```python
from build123d import *

# Parameters (mm, degrees)
F0_R     = 15
F0_R_2   = 5
F0_R_3   = 25
F1_DEPTH = 25


with BuildPart() as f1:
    # F0 (on Top) → F1 (new body)
    with BuildSketch(Plane.XY):
        with BuildLine():
            Line((-70.938008, -68.265357), (-67.75825, -73.265357))
            Line((-67.75825, -73.265357), (45.419062, -73.265357))
            Line((45.419062, -73.265357), (49.061992, -68.265357))
            Line((49.061992, -68.265357), (49.061992, -53.265357))
            Line((49.061992, -53.265357), (89.061992, -53.265357))
            Line((89.061992, -53.265357), (89.061992, 21.734643))
            ThreePointArc((89.061992, 21.734643), (81.739661, 39.412313), (64.061992, 46.734643))
            Line((64.061992, 46.734643), (-86.938008, 46.734643))
            Line((-86.938008, 46.734643), (-110.938008, 34.734643))
            Line((-110.938008, 34.734643), (-110.938008, -53.265357))
            Line((-110.938008, -53.265357), (-70.938008, -53.265357))
            Line((-70.938008, -53.265357), (-70.938008, -68.265357))
        make_face()
        with Locations((-80.938008, -23.265357)):
            Circle(F0_R, mode=Mode.SUBTRACT)
        with Locations((69.061992, -38.265357)):
            Circle(F0_R_2, mode=Mode.SUBTRACT)
        with Locations((-15.938008, 16.734643)):
            Circle(F0_R_3, mode=Mode.SUBTRACT)
    extrude(amount=F1_DEPTH)


solid = f1.part
```
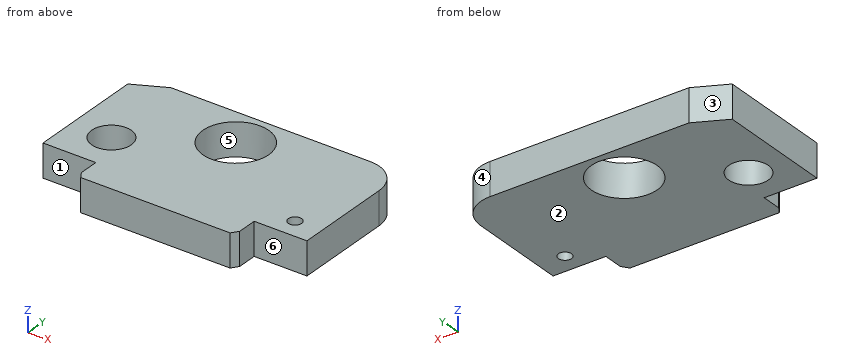
Work out the finished part from the listing and answer in its coordinate system (mm). Face numbers are marked on the shaded views. A direction names the side the tool comes from. Give positions to 0.01 mm unless a question says otherwise; leave off trailing zeros. Loops run counter-clockwise (first coordinate to the right, second up) from the corner with the lowest first, then second, coordinate; pieces in that order, holes last. Notation, with made-up numbers: (44.5, -15) -> (88.5, -15) arc R13 ccw to (88.5, -4) -> close; hole circle Ø3 at (14.5, 58.5). An arc over 180 degrees is marked (long way). Put each result on its own line as item: value. Start each with the question number.
Item 1: The part is cut by section B-B (z = 6.25). Give the vertices of the cut face in (x, y), then the cut area to 3 significant figures.
Item 2: Each of these flat-tipped pins is pushed along its axis until it touches: P1, Ø7.5, axis at y = -60.5, z = 11, coming from the +X side; P2, Ø7.5, axis at x = 73, z = 12.5, coming from the -Y side. Where does it stop, or does it pass through?
Item 3: The mould has two halves that part along X. Classify the marked faces 3, 4, 5 and 6: released by +X, released by -X, zero draft, split by the parting line, or undercut.
Item 4: Find the intervals of material crossed by L1, parallel to X at y = -17.5, z = 14.5; L2, parallel to X at y = 39.5, z = 8.75; L3, parallel to X at y = -37, z = 16, in increasing order. Write a range as [from, to].
Item 5: The part is cut by section C-C (x = -27.5). Give the vertices of the cut face in (y, z).
Item 6: The part is cut by section D-D (y = -64). Give the vertices of the cut face in (x, z).
Item 7: Which of the six approach directions +Z, -Z, +X, -X, +Y, -Y give full straight-line access (tool end or side, diameter ignored) to the marked faces 1 and 2?
Item 8: The part is cut by section A-A (y = -6). Give the vertices of the cut face in (x, z).
Answers below:
1. outline: (-110.94, -53.27) -> (-70.94, -53.27) -> (-70.94, -68.27) -> (-67.76, -73.27) -> (45.42, -73.27) -> (49.06, -68.27) -> (49.06, -53.27) -> (89.06, -53.27) -> (89.06, 21.73) arc R25 ccw to (64.06, 46.73) -> (-86.94, 46.73) -> (-110.94, 34.73) -> close; hole circle Ø30 at (-80.94, -23.27); hole circle Ø50 at (-15.94, 16.73); hole circle Ø10 at (69.06, -38.27)
1. area: 19,400 mm2
2. P1: x = 49.06
2. P2: y = -53.27
3. face 3: released by -X
3. face 4: released by +X
3. face 5: undercut
3. face 6: zero draft
4. L1: [-110.94, -94.79], [-67.09, 89.06]
4. L2: [-101.41, -26.27], [-5.61, 81.65]
4. L3: [-110.94, -86.97], [-74.91, 64.22], [73.9, 89.06]
5. outline: (-73.27, 0) -> (-5.43, 0) -> (-5.43, 25) -> (-73.27, 25) -> close; (38.9, 0) -> (46.73, 0) -> (46.73, 25) -> (38.9, 25) -> close
6. outline: (-70.94, 0) -> (49.06, 0) -> (49.06, 25) -> (-70.94, 25) -> close
7. face 1: +Z, -Z, -X, -Y
7. face 2: -Z, +X, -X, +Y, -Y
8. outline: (-110.94, 0) -> (-26.34, 0) -> (-26.34, 25) -> (-110.94, 25) -> close; (-5.54, 0) -> (89.06, 0) -> (89.06, 25) -> (-5.54, 25) -> close
